```python
from build123d import *
from OCP.BRepAlgoAPI import BRepAlgoAPI_Cut
from OCP.TopTools import TopTools_ListOfShape

# Parameters (mm, degrees)
SKETCH1_W           = 40.66
SKETCH1_H           = 31.77
SKETCH1_R           = 1.75
BOSS_EXTRUDE1_DEPTH = 2
SKETCH2_W           = 16.18
SKETCH2_H           = 11.33
BOSS_EXTRUDE2_DEPTH = 21.95
SKETCH3_W           = 18.18
SKETCH3_H           = 13.33
SKETCH3_W_2         = 16.18
SKETCH3_H_2         = 11.33
BOSS_EXTRUDE3_DEPTH = 19.25
FILLET2_START       = -21.95
FILLET2_DEPTH       = 21.95
FILLET2_START_2     = 2
FILLET2_2_DEPTH     = 19.25
FILLET2_3_DEPTH     = 43.2
FILLET3_R           = 2


with BuildPart() as part:
    # Sketch1 → Boss-Extrude1 (new body)
    with BuildSketch(Plane.XY):
        Rectangle(SKETCH1_W, SKETCH1_H)
        with Locations((-15.555, 11.585)):
            Circle(SKETCH1_R, mode=Mode.SUBTRACT)
        with Locations((-15.555, -11.585)):
            Circle(SKETCH1_R, mode=Mode.SUBTRACT)
        with Locations((15.555, -11.585)):
            Circle(SKETCH1_R, mode=Mode.SUBTRACT)
        with Locations((15.555, 11.585)):
            Circle(SKETCH1_R, mode=Mode.SUBTRACT)
    extrude(amount=BOSS_EXTRUDE1_DEPTH)

    # Sketch2 → Boss-Extrude2 (add)
    with BuildSketch(Plane(origin=(0, 0, 0), x_dir=(-1, 0, 0), z_dir=(0, 0, -1))):
        Polygon((6.245, -6.665), (9.09, -6.665), (9.09, 6.665), (-9.09, 6.665), (-9.09, -6.665), (-6.245, -6.665), (-6.245, -8.835), (6.245, -8.835), align=None)
        Rectangle(SKETCH2_W, SKETCH2_H, mode=Mode.SUBTRACT)
    extrude(amount=BOSS_EXTRUDE2_DEPTH)

    # Sketch3 → Boss-Extrude3 (add)
    with BuildSketch(Plane.XY.offset(2)):
        Rectangle(SKETCH3_W, SKETCH3_H)
        Rectangle(SKETCH3_W_2, SKETCH3_H_2, mode=Mode.SUBTRACT)
    extrude(amount=BOSS_EXTRUDE3_DEPTH)


with BuildPart() as fillet2_tool:
    # Fillet2: read off the stored shape, not the designer's step
    # Fillet2 outline → Fillet2 (new body)
    with BuildSketch(Plane.XY.offset(FILLET2_START)):
        with BuildLine():
            Line((-9.09, -6.665), (-6.245, -6.665))
            ThreePointArc((-6.245, -6.665), (-8.265430992, -5.734799668), (-9.09, -3.669006842))
            Line((-9.09, -3.669006842), (-9.09, -6.665))
        make_face()
        with BuildLine():
            Line((-9.09, 6.665), (-9.09, 3.665))
            ThreePointArc((-9.09, 3.665), (-8.211320344, 5.786320344), (-6.09, 6.665))
            Line((-6.09, 6.665), (-9.09, 6.665))
        make_face()
        with BuildLine():
            Line((9.09, -6.665), (9.09, -3.669006842))
            ThreePointArc((9.09, -3.669006842), (8.265430992, -5.734799668), (6.245, -6.665))
            Line((6.245, -6.665), (9.09, -6.665))
        make_face()
        with BuildLine():
            Line((9.09, 6.665), (6.09, 6.665))
            ThreePointArc((6.09, 6.665), (8.211320344, 5.786320344), (9.09, 3.665))
            Line((9.09, 3.665), (9.09, 6.665))
        make_face()
    extrude(amount=FILLET2_DEPTH)


with BuildPart() as part_1:
    add(part.part)

    # Fillet2: cut by fillet2_tool, with a tolerance
    fillet2_stock = TopTools_ListOfShape()
    fillet2_stock.Append(part_1.part.wrapped)
    fillet2_tools = TopTools_ListOfShape()
    fillet2_tools.Append(fillet2_tool.part.wrapped)
    fillet2_cut = BRepAlgoAPI_Cut()
    fillet2_cut.SetArguments(fillet2_stock)
    fillet2_cut.SetTools(fillet2_tools)
    fillet2_cut.SetFuzzyValue(0.00001)
    fillet2_cut.Build()
    add(Compound.cast(fillet2_cut.Shape()).solids(), mode=Mode.REPLACE)


with BuildPart() as fillet2_2_tool:
    # Fillet2 2 outline → Fillet2 2 (new body)
    with BuildSketch(Plane.XY.offset(FILLET2_START_2)):
        with BuildLine():
            Line((-9.09, -6.665), (-6.09, -6.665))
            ThreePointArc((-6.09, -6.665), (-8.209903239, -5.787736503), (-9.089997324, -3.669006838))
            Line((-9.089997324, -3.669006838), (-9.09, -6.665))
        make_face()
        with BuildLine():
            ThreePointArc((9.089997324, -3.669006838), (8.209903239, -5.787736503), (6.09, -6.665))
            Line((6.09, -6.665), (9.09, -6.665))
            Line((9.09, -6.665), (9.089997324, -3.669006838))
        make_face()
        with BuildLine():
            Line((-9.09, 6.665), (-9.09, 3.665))
            ThreePointArc((-9.09, 3.665), (-8.211320344, 5.786320344), (-6.09, 6.665))
            Line((-6.09, 6.665), (-9.09, 6.665))
        make_face()
        with BuildLine():
            Line((9.09, 6.665), (6.09, 6.665))
            ThreePointArc((6.09, 6.665), (8.211320344, 5.786320344), (9.09, 3.665))
            Line((9.09, 3.665), (9.09, 6.665))
        make_face()
    extrude(amount=FILLET2_2_DEPTH)


with BuildPart() as part_2:
    add(part_1.part)

    # Fillet2 2: cut by fillet2_2_tool, with a tolerance
    fillet2_2_stock = TopTools_ListOfShape()
    fillet2_2_stock.Append(part_2.part.wrapped)
    fillet2_2_tools = TopTools_ListOfShape()
    fillet2_2_tools.Append(fillet2_2_tool.part.wrapped)
    fillet2_2_cut = BRepAlgoAPI_Cut()
    fillet2_2_cut.SetArguments(fillet2_2_stock)
    fillet2_2_cut.SetTools(fillet2_2_tools)
    fillet2_2_cut.SetFuzzyValue(0.00001)
    fillet2_2_cut.Build()
    add(Compound.cast(fillet2_2_cut.Shape()).solids(), mode=Mode.REPLACE)


with BuildPart() as fillet2_3_tool:
    # Fillet2 3 outline → Fillet2 3 (new body)
    with BuildSketch(Plane.XY.offset(FILLET2_START)):
        with BuildLine():
            Line((-8.09, -5.665), (-5.09, -5.665))
            ThreePointArc((-5.09, -5.665), (-7.211320344, -4.786320344), (-8.09, -2.665))
            Line((-8.09, -2.665), (-8.09, -5.665))
        make_face()
        with BuildLine():
            ThreePointArc((8.09, -2.665), (7.211320344, -4.786320344), (5.09, -5.665))
            Line((5.09, -5.665), (8.09, -5.665))
            Line((8.09, -5.665), (8.09, -2.665))
        make_face()
        with BuildLine():
            Line((-8.09, 5.665), (-8.09, 2.665))
            ThreePointArc((-8.09, 2.665), (-7.211320344, 4.786320344), (-5.09, 5.665))
            Line((-5.09, 5.665), (-8.09, 5.665))
        make_face()
        with BuildLine():
            ThreePointArc((5.09, 5.665), (7.211320344, 4.786320344), (8.09, 2.665))
            Line((8.09, 2.665), (8.09, 5.665))
            Line((8.09, 5.665), (5.09, 5.665))
        make_face()
    extrude(amount=FILLET2_3_DEPTH)


with BuildPart() as part_3:
    add(part_2.part)


with BuildPart() as part_4:
    # Fillet2 3: joined with fillet2_3_tool
    add(part_3.part.fuse(fillet2_3_tool.part, tol=0.00001))

    # Fillet3
    fillet3_edges = [part_4.edges().sort_by_distance(p)[0] for p in [
        (-20.33, 15.885, 1),
        (20.33, 15.885, 1),
        (20.33, -15.885, 1),
        (-20.33, -15.885, 1),
    ]]
    fillet(fillet3_edges, radius=FILLET3_R)


solid = part_4.part
```
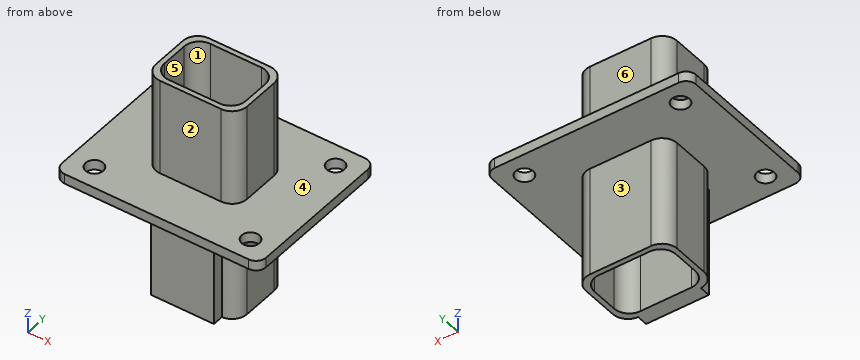
Work out the finished part from the listing and answer in its coordinate system (mm). Face numbers are marked on the shaded views. A direction names the side the tool comes from. Round coordinates to 2 decimals unless told otherwise and drop trailing zeros. Loops run counter-clockwise (first coordinate to the right, second up) from the corner with the lowest first, then second, coordinate; pieces in that order, holes last. Notation, with made-up numbers: (88.5, 2) -> (99.5, 2) arc R26 cw to (99.5, 27) -> close; hole circle Ø3 at (69, -26.5). An arc over 180 degrees is marked (long way). Write each question's results on one line, items separated by ' | '. Start each with the question number.
1. Section A-A (z = 12) is taken. Determine the outline of the cut face in (x, y) (3 decimals), plus the area to 3 significant figures.
2. For a pull along Y with two mould halves and no side action, classify the marked faces 4, 5 and 6 as +Y half, -Y half, draft (parallel to the pull), parting line (faces both ways), or undercut.
3. Given pin 1 Ø2.5 at (y, z) = (-8, -7) entering from -X (3 decimals); pin 2 Ø3 at (x, y) = (-15.555, -11.585) entering from -Z; pin 3 Ø1 at (x, y) = (0, -5.5) entering from -Z; pin 4 Ø8 at (x, z) = (11.5, 16) entering from -Y, each flat-ended and moving along its own axis, determine where each tip first touches the part or whether it passes through.
4. Find the intervals of material crossed by probe 1 along X at (y, z) = (2, -19.5); probe 2 along Y at (x, z) = (1.5, -14) (3 decimals); probe 3 along Z at (x, y) = (-15.5, -3), in increasing order. Write a range as from..to.
5. Section C-C (y = -1) is taken. Determine the outline of the cut face in (x, z), plus the area to 3 significant figures.
6. Section D-D (z = 1) is taken. Determine the outline of the cut face in (x, y) (3 decimals), plus the area to 3 significant figures.
7. Section B-B (x = -2) is taken. Determine the outline of the cut face in (y, z) (3 decimals).
8. A tool of negligible diameter and unlimited length cuts with its end or side. For the marked faces 1, 2 and 3, from which of +Z, -Z, +X, -X, +Y, -Y can it reach the whole face along a straight path? Write none if from no direction.
Evaluation:
1) outline: (-9.09, -3.669) arc R3 ccw to (-6.09, -6.665) -> (6.09, -6.665) arc R3 ccw to (9.09, -3.669) -> (9.09, 3.665) arc R3 ccw to (6.09, 6.665) -> (-6.09, 6.665) arc R3 ccw to (-9.09, 3.665) -> close; hole (-8.09, -2.665) arc R3 ccw to (-5.09, -5.665) -> (5.09, -5.665) arc R3 ccw to (8.09, -2.665) -> (8.09, 2.665) arc R3 ccw to (5.09, 5.665) -> (-5.09, 5.665) arc R3 ccw to (-8.09, 2.665) -> close | area: 59.0 mm2
2) face 4: draft | face 5: undercut | face 6: +Y half
3) pin 1: stops at x = -6.245 | pin 2: passes through | pin 3: stops at z = -21.95 | pin 4: stops at y = -6.31
4) probe 1: x = -9.09..-8.09, 8.09..9.09 | probe 2: y = -8.835..-5.665, 5.665..6.665 | probe 3: z = 0..2
5) outline: (-20.33, 0) -> (-9.09, 0) -> (-9.09, -21.95) -> (-8.09, -21.95) -> (-8.09, 0) -> (8.09, 0) -> (8.09, -21.95) -> (9.09, -21.95) -> (9.09, 0) -> (20.33, 0) -> (20.33, 2) -> (9.09, 2) -> (9.09, 21.25) -> (8.09, 21.25) -> (8.09, 2) -> (-8.09, 2) -> (-8.09, 21.25) -> (-9.09, 21.25) -> (-9.09, 2) -> (-20.33, 2) -> close | area: 164 mm2
6) outline: (-20.33, -13.885) arc R2 ccw to (-18.33, -15.885) -> (18.33, -15.885) arc R2 ccw to (20.33, -13.885) -> (20.33, 13.885) arc R2 ccw to (18.33, 15.885) -> (-18.33, 15.885) arc R2 ccw to (-20.33, 13.885) -> close; hole circle Ø3.5 at (-15.555, -11.585); hole circle Ø3.5 at (-15.555, 11.585); hole circle Ø3.5 at (15.555, -11.585); hole circle Ø3.5 at (15.555, 11.585) | area: 1,250 mm2
7) outline: (-15.885, 0) -> (-8.835, 0) -> (-8.835, -21.95) -> (-5.665, -21.95) -> (-5.665, 0) -> (5.665, 0) -> (5.665, -21.95) -> (6.665, -21.95) -> (6.665, 0) -> (15.885, 0) -> (15.885, 2) -> (6.665, 2) -> (6.665, 21.25) -> (5.665, 21.25) -> (5.665, 2) -> (-5.665, 2) -> (-5.665, 21.25) -> (-6.665, 21.25) -> (-6.665, 2) -> (-15.885, 2) -> close
8) face 1: +Z | face 2: +Z, +X, -X, -Y | face 3: -Z, +X, -X, +Y
